Verification items for this drawing (mm, ordinates from the low corner). A direction names the side the tool comes from. Give positions to 0.01 mm unless a question says otherwise; leave off trailing zeros. Order: outer loops, then holes, each group sorted by start corner. A loop starts at its lowest first (then second) coordinate and runs counter-clockwise, first axis right, second up. Notation, with made-up numbers: M 43,9.25 L 69,9.25 A18 cw 69,24.25 Z; hole C 62.25,66 d5. An arc over 180 degrees is marked long. One line per question, with ' | ' between items. Start each with the question number.
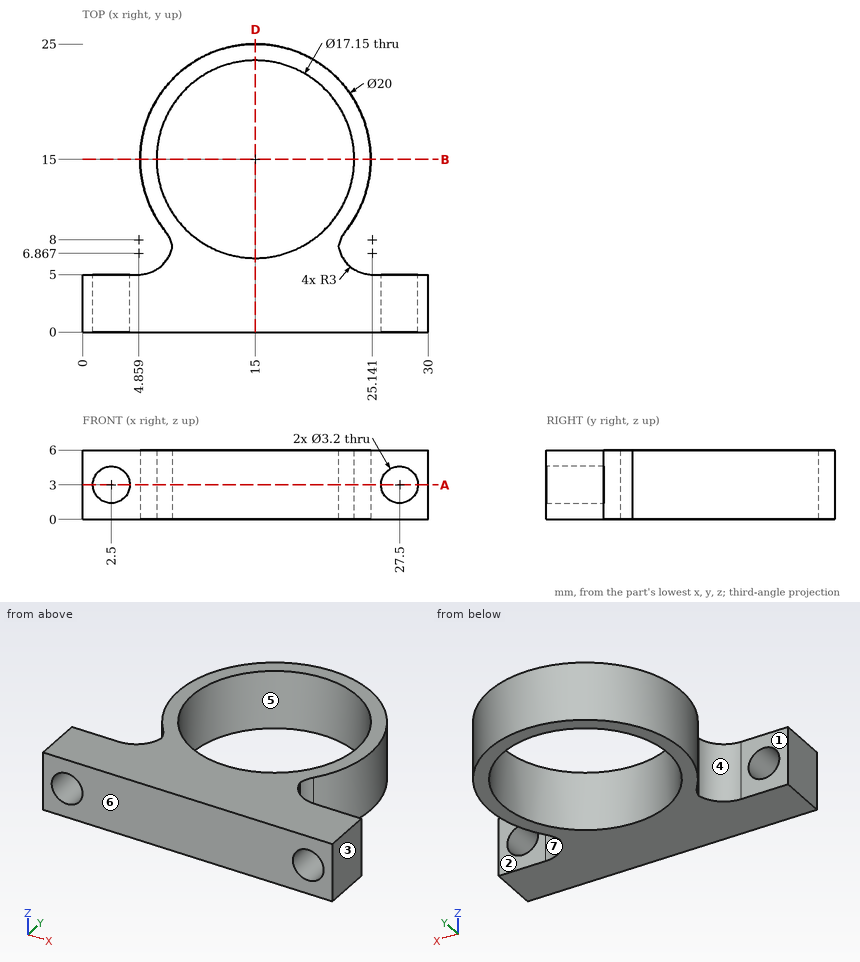
Item 1: Material ranges on line 1 along X through (y, z) = (1.05, 3); line 2 along Y through (x, z) = (15, 2.7) (1 decimal); line 3 along Y through (x, z) = (22.75, 1.85) (1 decimal), recorded low to high.
Item 2: Cross-section at A-A, the plane z = 3. State how many separate pieces and enclosed holes the cut face has.
Item 3: Depth check by flat-ended pin: pin 1 (3.5 mm diameter, centred on x = 2.5, z = 3, fed in from +Y); pin 2 (2.5 mm diameter, centred on x = 27.5, z = 3, fed in from +Y). Enter the tip coordinate at first touch or a pass-through.
Item 4: Cross-section at D-D, the plane x = 15. Record the cut outline in (y, z) (1 decimal).
Item 5: Set-up check for the marked faces 1, 2, 3 and 4: record each of +Z, -Z, +X, -X, +Y, -Y from which the full face is reachable in a straight line by a thin tool's end or side.
Item 6: Mould release check, pull along X, two halves, no side actions. Record for the marked faces 5, 6 and 7: released by +X, released by -X, zero draft, split by the parting line, or undercut.
Item 7: Cross-section at B-B, the plane y = 15. Record the cut outline in (x, z) (1 decimal).
Outcome:
1) line 1: x = 0 to 0.9, 4.1 to 25.9, 29.1 to 30 | line 2: y = 0 to 6.4, 23.6 to 25 | line 3: y = 0 to 6.2, 8.7 to 11.3, 18.7 to 21.3
2) separate pieces: 3 | enclosed holes: 1
3) pin 1: stops at y = 5 | pin 2: passes through
4) outline: M 0,0 L 6.4,0 L 6.4,6 L 0,6 Z; M 23.6,0 L 25,0 L 25,6 L 23.6,6 Z
5) face 1: +Z, -Z, -X, +Y | face 2: +Z, -Z, +X, +Y | face 3: +Z, -Z, +X, +Y, -Y | face 4: +Z, -Z, -X
6) face 5: undercut | face 6: zero draft | face 7: released by +X
7) outline: M 5,0 L 6.4,0 L 6.4,6 L 5,6 Z; M 23.6,0 L 25,0 L 25,6 L 23.6,6 Z
